from build123d import *

# Parameters (mm, degrees)
SKETCH_1_R          = 3
SKETCH_1_R_2        = 2.05
EXTRUDE_1_DEPTH     = 4
SKETCH_2_R          = 1.65
CUT_EXTRUDE_1_DEPTH = 5


with BuildPart() as part:
    # 草图1 → 凸台-拉伸1 (new body)
    with BuildSketch(Plane(origin=(0, 0, 0), x_dir=(0, 0, -1), z_dir=(1, 0, 0))):
        with BuildLine():
            Line((0, 6), (90, 6))
            ThreePointArc((90, 6), (96, 0), (90, -6))
            Line((90, -6), (0, -6))
            ThreePointArc((0, -6), (-6, 0), (0, 6))
        make_face()
        Circle(SKETCH_1_R, mode=Mode.SUBTRACT)
        with Locations((90, 0)):
            Circle(SKETCH_1_R_2, mode=Mode.SUBTRACT)
    extrude(amount=EXTRUDE_1_DEPTH)

    # 草图2 → 切除-拉伸1 (cut, through all)
    with BuildSketch(Plane(origin=(4, 0, 0), x_dir=(0, 0, -1), z_dir=(1, 0, 0))):
        with Locations((52, 0)):
            Circle(SKETCH_2_R)
    extrude(amount=-CUT_EXTRUDE_1_DEPTH, mode=Mode.SUBTRACT)


solid = part.part
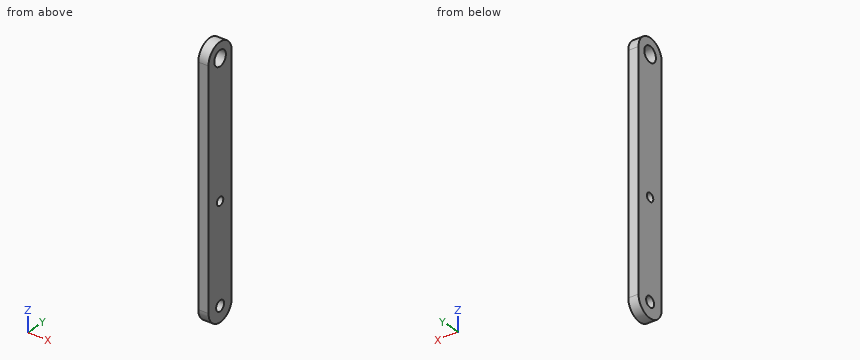
Could you check a few things on this model? Use its own coordinates, in mm. Give positions to 0.01 mm unless a question says otherwise; leave off trailing zeros. Write each loop counter-clockwise with the first axis right and the second up, starting at its lowest first coordinate (ties: lowest second). Pieces come first, ordered by that corner, then holes. Notation, with made-up numbers: (-37, -34.5) -> (16, -34.5) arc R31 cw to (16, 0.5) -> close; hole circle Ø10 at (66, 11). An arc over 180 degrees is marked (long way). Answer as a JSON object with one key per item and string values.
Q1. Suppose I cut it at A-A on z = -52. Write out the boundary of the cut face in (x, y), then the cut area to 3 significant figures.
Taken from the geometry:
{"outline": "(0, -6) -> (4, -6) -> (4, -1.65) -> (0, -1.65) -> close; (0, 1.65) -> (4, 1.65) -> (4, 6) -> (0, 6) -> close", "area": "34.8 mm²"}
Q2. Please list where these lines run through material, in increasing order: L1, parallel to Y at x = 2.5, z = -90; L2, parallel to Z at x = 0.25, y = -1.5; L3, parallel to Z at x = 0.55, y = 0.75.
Taken from the geometry:
{"L1": "y = -6 to -2.05, 2.05 to 6", "L2": "z = -95.81 to -91.4, -88.6 to -52.69, -51.31 to -2.6, 2.6 to 5.81", "L3": "z = -95.95 to -91.91, -88.09 to -53.47, -50.53 to -2.9, 2.9 to 5.95"}
Q3. Suppose I cut it at C-C on x = 1.75. Write out the boundary of the cut face in (y, z).
Taken from the geometry:
{"outline": "(-6, -90) arc R6 ccw to (6, -90) -> (6, 0) arc R6 ccw to (-6, 0) -> close; hole circle Ø6 at (0, 0); hole circle Ø4.1 at (0, -90); hole circle Ø3.3 at (0, -52)"}
Q4. Suppose I cut it at D-D on y = 4.5. Write out the boundary of the cut face in (x, z), then the cut area to 3 significant figures.
Taken from the geometry:
{"outline": "(0, -93.97) -> (4, -93.97) -> (4, 3.97) -> (0, 3.97) -> close", "area": "392 mm²"}
Q5. Suppose I cut it at B-B on y = 0. Write out the boundary of the cut face in (x, z).
Taken from the geometry:
{"outline": "(0, -96) -> (4, -96) -> (4, -92.05) -> (0, -92.05) -> close; (0, -87.95) -> (4, -87.95) -> (4, -53.65) -> (0, -53.65) -> close; (0, -50.35) -> (4, -50.35) -> (4, -3) -> (0, -3) -> close; (0, 3) -> (4, 3) -> (4, 6) -> (0, 6) -> close"}
Q6. Will this pin go through, and if not, where does the flat tip stop? pin 1 Ø5.5 at (y, z) = (0, 0) entering from +X.
Taken from the geometry:
{"pin 1": "passes through"}
